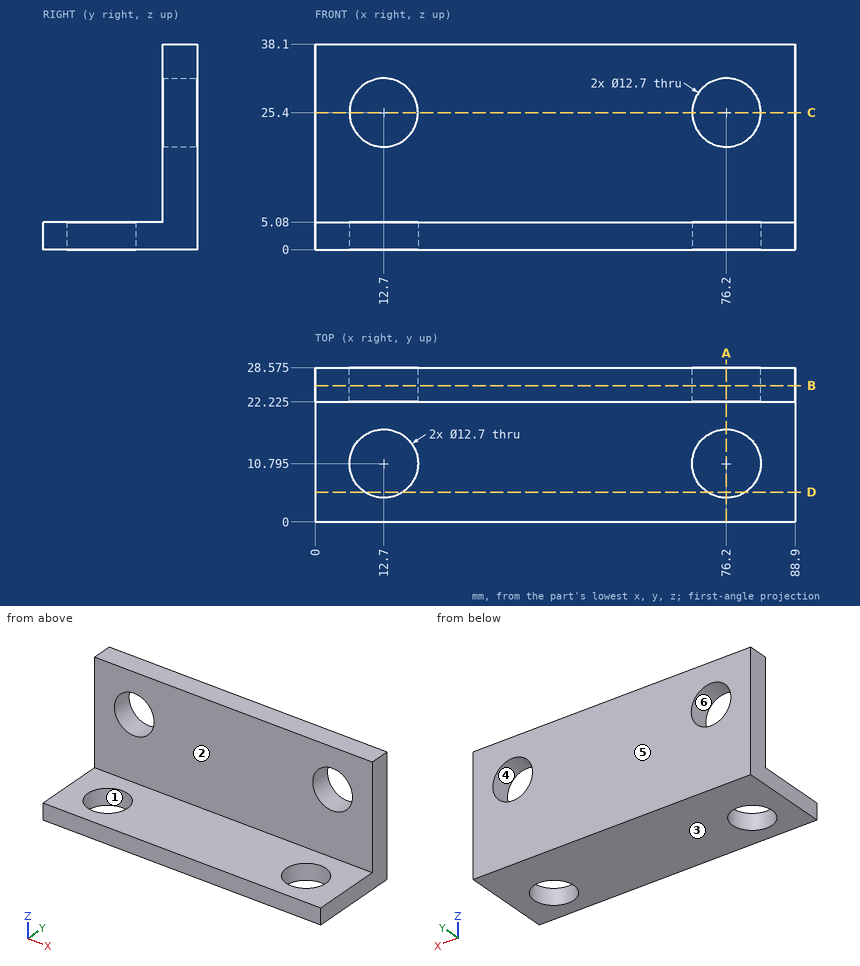
Geometry: see drawing. Coordinates: mm, zero at the bounding-box minimum. A direction names the side the tool comes from. Give positions to 0.01 mm unless a question says otherwise; leave off trailing zeros. Order: outer loops, then holes, each group sorted by start corner. A loop starts at its lowest first (then second) coordinate and runs counter-clockwise, first axis right, second up. Notation, with made-up numbers: (59.25, -27) - (81.25, -27) arc R36 ccw to (81.25, 12) - close; hole circle Ø8 at (36.25, 67). An arc over 180 degrees is marked (long way). One line per item, written item: value.
1. Cut plane C-C, the plane z = 25.4. Output: boundary loops of the cut face in (x, y) (3 decimals), and give its area (3 significant figures).
Determined:
outline: (0, 22.225) - (6.35, 22.225) - (6.35, 28.575) - (0, 28.575) - close; (19.05, 22.225) - (69.85, 22.225) - (69.85, 28.575) - (19.05, 28.575) - close; (82.55, 22.225) - (88.9, 22.225) - (88.9, 28.575) - (82.55, 28.575) - close
area: 403 mm2
2. Line query: probe 1 along X at (y, z) = (27.75, 25.5); probe 2 along Y at (x, z) = (76.2, 1.8) (3 decimals); probe 3 along X at (y, z) = (13, 2). Output: solid intervals per line, ascending.
Determined:
probe 1: 0 to 6.35, 19.05 to 69.85, 82.55 to 88.9
probe 2: 0 to 4.445, 17.145 to 28.575
probe 3: 0 to 6.75, 18.65 to 70.25, 82.15 to 88.9
3. Draft query along Z for the marked faces 3, 4, 5 and 6. Return one class per face: released by +Z, released by -Z, zero draft, split by the parting line, or undercut.
Determined:
face 3: released by -Z
face 4: undercut
face 5: zero draft
face 6: undercut
4. Cut plane A-A, the plane x = 76.2. Output: boundary loops of the cut face in (y, z) (3 decimals).
Determined:
outline: (0, 0) - (4.445, 0) - (4.445, 5.08) - (0, 5.08) - close; (17.145, 0) - (28.575, 0) - (28.575, 19.05) - (22.225, 19.05) - (22.225, 5.08) - (17.145, 5.08) - close; (22.225, 31.75) - (28.575, 31.75) - (28.575, 38.1) - (22.225, 38.1) - close
5. Cut plane D-D, the plane y = 5.5. Output: boundary loops of the cut face in (x, z).
Determined:
outline: (0, 0) - (9.19, 0) - (9.19, 5.08) - (0, 5.08) - close; (16.21, 0) - (72.69, 0) - (72.69, 5.08) - (16.21, 5.08) - close; (79.71, 0) - (88.9, 0) - (88.9, 5.08) - (79.71, 5.08) - close
6. Cut plane B-B, the plane y = 25.25. Output: boundary loops of the cut face in (x, z).
Determined:
outline: (0, 0) - (88.9, 0) - (88.9, 38.1) - (0, 38.1) - close; hole circle Ø12.7 at (12.7, 25.4); hole circle Ø12.7 at (76.2, 25.4)
7. Reachability of the marked faces 1 and 2 from +Z, -Z, +X, -X, +Y, -Y: full face, straight path, thin tool, end or side. Return the list, or none.
Determined:
face 1: +Z, -Z
face 2: +Z, +X, -X, -Y
8. Pin query (flat end, axial travel): pin 1 Ø11 at (x, y) = (23, 8) entering from +Z; pin 2 Ø10 at (x, z) = (65.5, 24) entering from -Y (3 decimals). Return the tip coordinate at first contact, or that it passes through.
Determined:
pin 1: z = 5.08
pin 2: y = 22.225
